The figure shows three views and two pictorial views of one solid part (mm, origin at its lowest corner). Answer the questions. Give positions to 0.01 mm unless a question says otherwise; leave off trailing zeros. Write each loop counter-clockwise with the first axis right and the second up, starting at its lowest first coordinate (ties: lowest second). Pieces come first, ordered by that corner, then holes. Notation, with made-up numbers: M 78,-19.5 L 106,-19.5 A34 cw 106,11.5 Z; hole C 73,59.25 d10. An arc over 180 degrees is marked long. Answer as CSV lines item,"result". Start each with the question number.
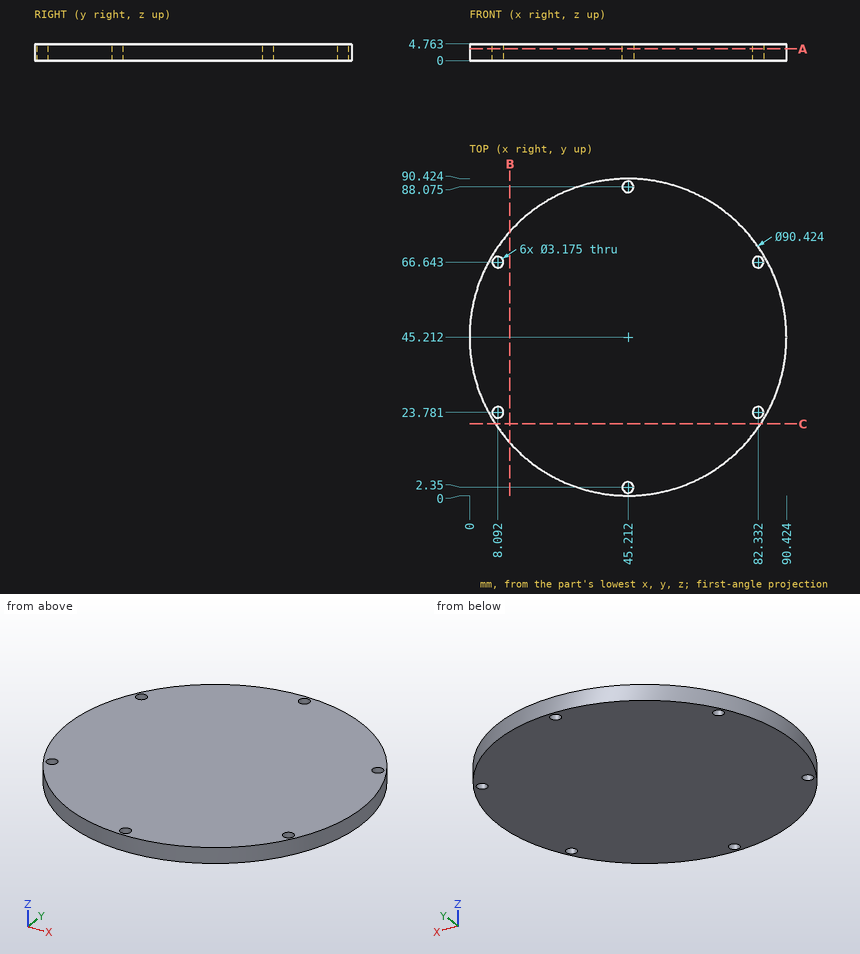
1. Given pin 1 (2 mm diameter, centred on y = 79.5, z = 0.5, fed in from -X); pin 2 (1.5 mm diameter, centred on x = 72.5, z = 3.5, fed in from +Y) (1 decimal); pin 3 (3 mm diameter, centred on x = 8.09, y = 23.78, fed in from -Z), each flat-ended and moving along its own axis, determine where each tip first touches the part or whether it passes through.
2. Find section B-B on x = 11.5. Determine the outline of the cut face in (y, z) (1 decimal).
3. Find the intervals of material crossed by line 1 (Y direction, x = 81, z = 2.35) (1 decimal); line 2 (X direction, y = 45.5, z = 1.4); line 3 (X direction, y = 67, z = 4.2) (1 decimal), in increasing order. Write a range as [from, to].
4. Find section C-C on y = 20.5. Determine the outline of the cut face in (x, z).
5. Find section A-A on z = 3.35. State how many separate pieces and enclosed holes the cut face has, then the cut area to 3 significant figures.
Computed:
1,pin 1,"stops at x = 14.62"
1,pin 2,"stops at y = 81.8"
1,pin 3,"passes through"
2,outline,"M 15.1,0 L 75.3,0 L 75.3,4.8 L 15.1,4.8 Z"
3,line 1,"y = [17.6, 22.9], [24.6, 65.8], [67.5, 72.8]"
3,line 2,"x = [0, 90.42]"
3,line 3,"x = [5.6, 6.5], [9.6, 80.8], [83.9, 84.8]"
4,outline,"M 7.35,0 L 83.07,0 L 83.07,4.76 L 7.35,4.76 Z"
5,separate pieces,"1"
5,enclosed holes,"6"
5,area,"6,370 mm^2"
